Autodesk Inventor part; units mm, degrees
ref_plane "YZ Plane" through (0, 0, 0) normal (1, 0, 0) x (0, 1, 0)
ref_plane "XZ Plane" through (0, 0, 0) normal (0, 1, 0) x (-1, 0, 0)
ref_plane "XY Plane" through (0, 0, 0) normal (0, 0, 1) x (1, 0, 0)
sketch "スケッチ1" plane through (0, 0, 0) normal (0, 0, 1) x (1, 0, 0)
  line L0 (-50, -50) -> (50, -50)
  line L1 (50, -50) -> (50, 50)
  line L2 (50, 50) -> (-50, 50)
  line L3 (-50, 50) -> (-50, -50)
  line L4 (-50, -50) -> (50, 50) construction
  line L5 (50, -50) -> (-50, 50) construction
  line L6 (35, 35) -> (40, 40) construction
  line L7 (31.4645, 38.5355) -> (36.4645, 43.5355)
  line L8 (43.5355, 36.4645) -> (38.5355, 31.4645)
  arc A0 (31.4645, 38.5355) -> (38.5355, 31.4645) centre (35, 35) ccw
  arc A1 (43.5355, 36.4645) -> (36.4645, 43.5355) centre (40, 40) ccw
  line L9 (-50, 0) -> (50, 0) construction
  line L10 (0, 50) -> (0, -50) construction
  line L11 (-35, 35) -> (-40, 40) construction
  line L12 (-31.4645, 38.5355) -> (-36.4645, 43.5355)
  line L13 (-43.5355, 36.4645) -> (-38.5355, 31.4645)
  arc A2 (-38.5355, 31.4645) -> (-31.4645, 38.5355) centre (-35, 35) ccw
  arc A3 (-36.4645, 43.5355) -> (-43.5355, 36.4645) centre (-40, 40) ccw
  line L14 (35, -35) -> (40, -40) construction
  line L15 (31.4645, -38.5355) -> (36.4645, -43.5355)
  line L16 (43.5355, -36.4645) -> (38.5355, -31.4645)
  arc A4 (38.5355, -31.4645) -> (31.4645, -38.5355) centre (35, -35) ccw
  arc A5 (36.4645, -43.5355) -> (43.5355, -36.4645) centre (40, -40) ccw
  arc A6 (-31.4645, -38.5355) -> (-38.5355, -31.4645) centre (-35, -35) ccw
  line L17 (-43.5355, -36.4645) -> (-38.5355, -31.4645)
  line L18 (-35, -35) -> (-40, -40) construction
  arc A7 (-43.5355, -36.4645) -> (-36.4645, -43.5355) centre (-40, -40) ccw
  line L19 (-31.4645, -38.5355) -> (-36.4645, -43.5355)
  point P0 (0, 0)
  point P1 (37.5, 37.5)
  point P2 (-37.5, 37.5)
  point P3 (37.5, -37.5)
  point P4 (-37.5, -37.5)
  dimension "d0" = 100
  dimension "d1" = 100
  dimension "d2" = 10
  dimension "d3" = 15
  dimension "d4" = 5
extrude "押し出し1" add sketch "スケッチ1" along normal blind 5
fillet "フィレット1" radius 10 4 edges at (50, 50, 2.5) (50, -50, 2.5) (-50, -50, 2.5) (-50, 50, 2.5)
sketch "スケッチ2" plane through (0, 0, 5) normal (0, 0, 1) x (1, 0, 0)
  circle A0 centre (0, 0) radius 12
  dimension "d8" = 24
extrude "押し出し2" add sketch "スケッチ2" along normal blind 20
properties part number "自由輪パーツ2"
Work out the finished part from the listing and answer in its coordinate system (mm). A direction names the side the tool comes from. Give positions to 0.01 mm unless a question says otherwise; leave off trailing zeros. Write each loop counter-clockwise with the first axis right and the second up, starting at its lowest first coordinate (ties: lowest second). Pieces come first, ordered by that corner, then holes. Notation, with made-up numbers: (28.25, 57) - (44.25, 57) arc R11 ccw to (44.25, 76) - close; hole circle Ø3 at (61, 32.25). An arc over 180 degrees is marked (long way). One line per item, written item: value. Start each with the question number.
1. Find section D-D (z = 13.5). Write down the section's boundary in (x, y).
2. Find section A-A (x = -35). Write down the section's boundary in (y, z), then the cut area to 3 significant figures.
3. For a pull along X with two mould halves and no side action, classify faces 1 (the flat face through (-50, 1, 2)), 2 (the flat face through (-1, -50, 2)), 3 (the flat face through (-41.07, 34, 2.46)) as +X half, -X half, draft (parallel to the pull), parting line (faces both ways), or undercut.
4. Find section C-C (y = 0). Write down the section's boundary in (x, z).
5. Consider probe 1 along Z at (x, y) = (-13.5, 9.5); probe 2 along X at (y, z) = (34.5, 4.5); probe 3 along Y at (x, z) = (37.5, 2). Determine where each line is inside the solid, lowest interval first.
6. Given pin 1 (8 mm diameter, centred on x = 2.5, y = -32.5, fed in from +Z); pin 2 (12 mm diameter, centred on x = 0.5, z = 18.5, fed in from +Y), each flat-ended and moving along its own axis, determine where each tip first touches the part or whether it passes through.
7. For faces 4 (the cylindrical face through (-11.99, -0.53, 14.86)), 5 (the cylindrical face through (-47.15, -46.99, 2.54)), 6 (the flat face through (-33.93, -41, 2.46)), determine the directions among +Z, -Z, +X, -X, +Y, -Y from which every point of the face is accessible in a straight line to the end or side of a thin tool.
Geometry results:
1. outline: circle Ø24 at (0, 0)
2. outline: (-50, 0) - (-42.07, 0) - (-42.07, 5) - (-50, 5) - close; (-30, 0) - (30, 0) - (30, 5) - (-30, 5) - close; (42.07, 0) - (50, 0) - (50, 5) - (42.07, 5) - close
2. area: 379 mm2
3. face 1: -X half
3. face 2: draft
3. face 3: undercut
4. outline: (-50, 0) - (50, 0) - (50, 5) - (12, 5) - (12, 25) - (-12, 25) - (-12, 5) - (-50, 5) - close
5. probe 1: 0 to 5
5. probe 2: -50 to -41.57, -30.03 to 30.03, 41.57 to 50
5. probe 3: -50 to -44.33, -30.67 to 30.67, 44.33 to 50
6. pin 1: z = 5
6. pin 2: y = 12
7. face 4: +Z
7. face 5: +Z, -Z, -X, -Y
7. face 6: +Z, -Z
